from build123d import *

# Parameters (mm, degrees)
SKETCH1_W           = 40.5
SKETCH1_H           = 16
SKETCH1_R           = 1.35
BOSS_EXTRUDE1_DEPTH = 12
BOSS_EXTRUDE2_START = 2
BOSS_EXTRUDE2_DEPTH = 10
SKETCH3_R           = 2.85
BOSS_EXTRUDE3_DEPTH = 12
FILLET2_R           = 5


with BuildPart() as part:
    # Sketch1 → Boss-Extrude1 (new body)
    with BuildSketch(Plane(origin=(0, 0, 0), x_dir=(1, 0, 0), z_dir=(0, 1, 0))):
        Rectangle(SKETCH1_W, SKETCH1_H)
        with Locations(Location((-17.25, 5, 0), (0, 0, 270))):
            Circle(SKETCH1_R, mode=Mode.SUBTRACT)
        with BuildLine():
            Line((-14.421572875, 6), (-1.078427125, 6))
            ThreePointArc((-1.078427125, 6), (1.75, 2), (4.578427125, 6))
            Line((4.578427125, 6), (18.25, 6))
            Line((18.25, 6), (18.25, -6))
            Line((18.25, -6), (-18.25, -6))
            Line((-18.25, -6), (-18.25, 2.171572875))
            ThreePointArc((-18.25, 2.171572875), (-15.128679656, 2.878679656), (-14.421572875, 6))
        make_face(mode=Mode.SUBTRACT)
        with Locations(Location((1.75, 5, 0), (0, 0, 270))):
            Circle(SKETCH1_R, mode=Mode.SUBTRACT)
    extrude(amount=BOSS_EXTRUDE1_DEPTH)

    # Sketch1<3> → Boss-Extrude2 (add)
    with BuildSketch(Plane(origin=(0, 0, 0), x_dir=(1, 0, 0), z_dir=(0, 1, 0)).offset(BOSS_EXTRUDE2_START)):
        with BuildLine():
            ThreePointArc((-14.25, 5), (-15.517949192, 2.550510257), (-18.25, 2.171572875))
            Line((-18.25, 2.171572875), (-18.25, -6))
            Line((-18.25, -6), (18.25, -6))
            Line((18.25, -6), (18.25, 6))
            Line((18.25, 6), (4.578427125, 6))
            ThreePointArc((4.578427125, 6), (4.706795679, 5.507305936), (4.75, 5))
            ThreePointArc((4.75, 5), (1.242694064, 2.043204321), (-1.078427125, 6))
            Line((-1.078427125, 6), (-14.421572875, 6))
            ThreePointArc((-14.421572875, 6), (-14.293204321, 5.507305936), (-14.25, 5))
        make_face()
    extrude(amount=BOSS_EXTRUDE2_DEPTH)

    # Sketch3 → Boss-Extrude3 (add)
    with BuildSketch(Plane(origin=(20.25, 0, 0), x_dir=(0, 0, -1), z_dir=(1, 0, 0))):
        with BuildLine():
            ThreePointArc((13.999999499, 12.000000501), (20.00000025, 6.000000501), (14, 0))
            Line((14, 0), (8, 0))
            Line((8, 0), (8, 12))
            Line((8, 12), (13.999999499, 12.000000501))
        make_face()
        with Locations((14, 6.000000501)):
            Circle(SKETCH3_R, mode=Mode.SUBTRACT)
    extrude(amount=-BOSS_EXTRUDE3_DEPTH)

    # Fillet2
    # the kernel refuses this fillet: 5 mm, written as the material it takes off along each edge
    with BuildSketch(Plane(origin=(-20.25, 12, -20.5), x_dir=(1, 0, 0), z_dir=(0, 0, 1))) as fillet2_piece_1:
        with BuildLine():
            CenterArc((FILLET2_R, -FILLET2_R), FILLET2_R, 90, 90)
            Line((0, -FILLET2_R), (0, 0))
            Line((0, 0), (FILLET2_R, 0))
        make_face()
    extrude(amount=41, mode=Mode.SUBTRACT)
    with BuildSketch(Plane(origin=(8.25, 12, -8), x_dir=(0, -1, 0), z_dir=(-1, 0, 0))) as fillet2_piece_2:
        with BuildLine():
            CenterArc((FILLET2_R, FILLET2_R), FILLET2_R, 180, 90)
            Line((0, FILLET2_R), (0, 0))
            Line((0, 0), (FILLET2_R, 0))
        make_face()
    extrude(amount=41, mode=Mode.SUBTRACT)
    with BuildSketch(Plane(origin=(-32.75, 12, 8), x_dir=(0, -1, 0), z_dir=(1, 0, 0))) as fillet2_piece_3:
        with BuildLine():
            CenterArc((FILLET2_R, FILLET2_R), FILLET2_R, 180, 90)
            Line((0, FILLET2_R), (0, 0))
            Line((0, 0), (FILLET2_R, 0))
        make_face()
    extrude(amount=65.5, mode=Mode.SUBTRACT)


solid = part.part
The listing builds one solid part. Answer for the finished solid, in the listing's coordinates (mm). A direction names the side the tool comes from. Give positions to 0.01 mm unless a question says otherwise; leave off trailing zeros. Write each loop counter-clockwise with the first axis right and the second up, starting at its lowest first coordinate (ties: lowest second). Pieces come first, ordered by that corner, then holes. Notation, with made-up numbers: (-18.75, 32) - (29.25, 32) arc R23 ccw to (29.25, 62) - close; hole circle Ø2 at (3, 80). An arc over 180 degrees is marked (long way). Use a Markdown table: item, result.
1. Find the intervals of material crossed by probe 1 along X at (y, z) = (6.5, -5); probe 2 along X at (y, z) = (9.5, -5); probe 3 along Z at (x, y) = (-17.25, 3.5), in increasing order. Write a range as from..to.
Values follow:
| item | result |
|---|---|
| probe 1 | x = -20.25..-18.6, -15.9..0.4, 3.1..20.25 |
| probe 2 | x = -19.58..-18.6, -15.9..0.4, 3.1..20.25 |
| probe 3 | z = -8..-6.35, -3.65..8 |
2. Section D-D on z = -5 is taken. Write down the section's boundary in (x, y), plus the area to 3 significant figures.
Values follow:
| item | result |
|---|---|
| outline | (-20.25, 0) - (-18.6, 0) - (-18.6, 10.71) arc R5 ccw to (-20.25, 7) - close; (-15.9, 0) - (-14.25, 0) - (-14.25, 2) - (-1.25, 2) - (-1.25, 0) - (0.4, 0) - (0.4, 11.58) - (-15.9, 11.58) - close; (3.1, 0) - (4.75, 0) - (4.75, 2) - (18.25, 2) - (18.25, 0) - (20.25, 0) - (20.25, 12) - (8.25, 12) - (8.25, 11.58) - (3.1, 11.58) - close |
| area | 355 mm² |
3. For a pull along Z with two mould halves and no side action, classify faces 1 (the cylindrical face through (14, 6, -20)), 2 (the flat face through (0, 1, 6)), 3 (the flat face through (20.25, 6, -6)) as released by +Z, released by -Z, zero draft, split by the parting line, or undercut.
Values follow:
| item | result |
|---|---|
| face 1 | released by -Z |
| face 2 | undercut |
| face 3 | zero draft |
4. A tool of negligible diameter and unlimited length cuts with its end or side. For faces 4 (the flat face through (11, 1, -6)), 5 (the flat face through (-6, 3, -8)), 6 (the cylindrical face through (-6, 11, -6)), from which of +Z, -Z, +X, -X, +Y, -Y can it reach the whole face along a straight path? Write none if from no direction.
Values follow:
| item | result |
|---|---|
| face 4 | -Y |
| face 5 | -Z, -X, +Y, -Y |
| face 6 | -Z, -X, +Y |
5. Section A-A on y = 6 is taken. Write down the section's boundary in (x, z), plus the area to 3 significant figures.
Values follow:
| item | result |
|---|---|
| outline | (-20.25, -8) - (8.25, -8) - (8.25, -11.15) - (20.25, -11.15) - (20.25, 8) - (-20.25, 8) - close; (8.25, -20) - (20.25, -20) - (20.25, -16.85) - (8.25, -16.85) - close; hole circle Ø2.7 at (-17.25, -5); hole circle Ø2.7 at (1.75, -5) |
| area | 712 mm² |
6. Each of these flat-tipped pins is pushed along its axis until it touches: P1, Ø1, axis at x = 6, y = 0.5, coming from the -Z side; P2, Ø3, axis at x = -17.25, z = -5, coming from the +Y side; P3, Ø10, axis at x = -4.5, z = -14.5, coming from the -Y side; P4, Ø8, axis at x = 10, z = 0.5, coming from the -Y side. Where does it stop, or does it pass through?
Values follow:
| item | result |
|---|---|
| P1 | stops at z = -8 |
| P2 | stops at y = 11.91 |
| P3 | passes through |
| P4 | stops at y = 2 |
7. Section B-B on x = 17.5 is taken. Write down the section's boundary in (y, z), plus the area to 3 significant figures.
Values follow:
| item | result |
|---|---|
| outline | (0, -14) arc R6 ccw to (12, -14) - (12, 3) arc R5 ccw to (7, 8) - (0, 8) - (0, 6) - (2, 6) - (2, -6) - (0, -6) - close; hole circle Ø5.7 at (6, -14) |
| area | 266 mm² |
8. Section C-C on x = -12.5 is taken. Write down the section's boundary in (y, z).
Values follow:
| item | result |
|---|---|
| outline | (0, -8) - (7, -8) arc R5 ccw to (12, -3) - (12, 3) arc R5 ccw to (7, 8) - (0, 8) - (0, 6) - (2, 6) - (2, -6) - (0, -6) - close |
